Part print with two shaded views. Sizes in mm from the minimum x, y, z corner. A direction names the side the tool comes from. Round coordinates to 2 decimals unless told otherwise and drop trailing zeros. Loops run counter-clockwise (first coordinate to the right, second up) from the corner with the lowest first, then second, coordinate; pieces in that order, holes last. Notation, with made-up numbers: M 9,66 L 54,66 A15 cw 54,72 Z; hole C 25.25,25.5 d2. An arc over 180 degrees is marked long. Answer as CSV lines item,"result". Start each with the question number.
Item 1: Which spindle directions (+Z, -Z, +X, -X, +Y, -Y) get a long thin tool onto all of the face, cutting with end or side? Do the marked faces 1 and 2. Say none if no direction does.
Item 2: Mould opens along Y. For the marked faces 3, 4, 5 and 6 say: pulls with the +Y half, pulls with the -Y half, needs draft (parallel to the pull), parting line crosses it, or undercut.
Item 3: Band-saw the part on C-C (z = 8.5). Give the cut face in (x, y), and give its area (3 significant figures).
Item 4: Band-saw the part on A-A (y = 66). Give the cut face in (x, z).
Item 5: Band-saw the part on B-B (x = 5). Give the cut face in (y, z).
Item 6: Wall check: line 1 (Y direction, x = 77, z = 15.25); line 2 (X direction, y = 46, z = 10.25); line 3 (Y direction, x = 30.5, z = 2.25). Give the ranges that are in metal, low to high.
Item 7: Band-saw the part on D-D (x = 68.5). Give the cut face in (y, z).
Item 8: Drop a flat-ended pin along its axis: pin 1 Ø3.5 at (x, y) = (5, 5) entering from +Z. Give the stop position or say it passes through.
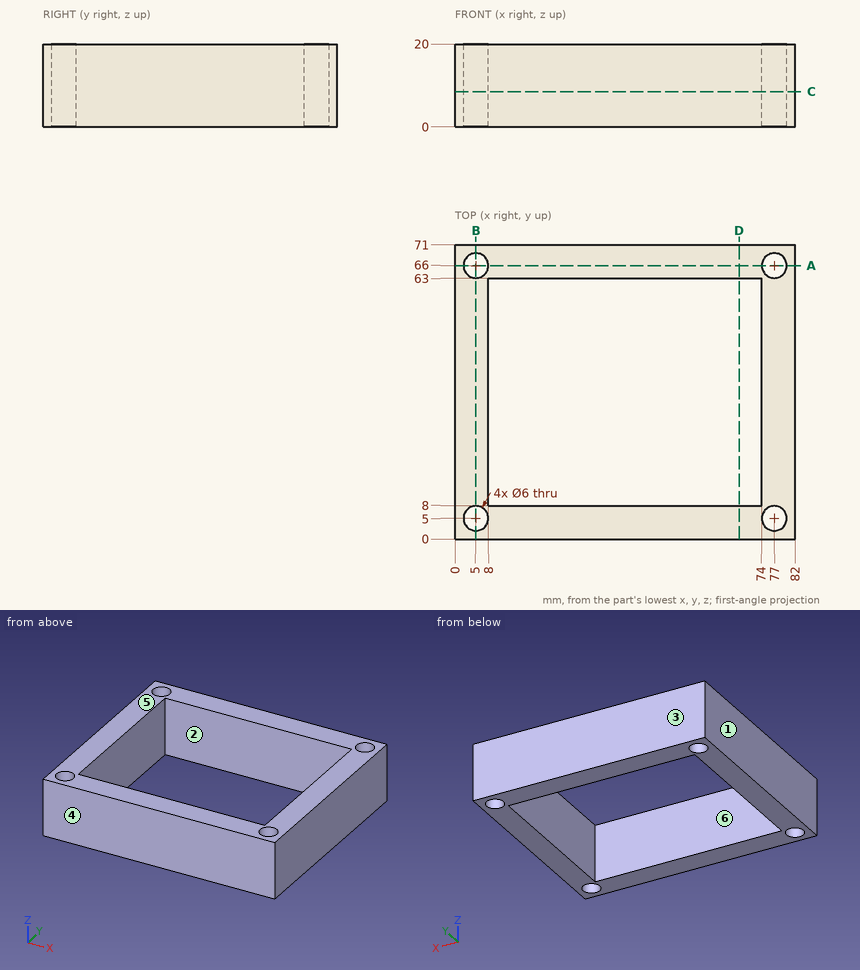
Answer block:
1,face 1,"+Z, -Z, -X, +Y, -Y"
1,face 2,"+Z, -Z"
2,face 3,"pulls with the +Y half"
2,face 4,"pulls with the -Y half"
2,face 5,"needs draft"
2,face 6,"undercut"
3,outline,"M 0,0 L 82,0 L 82,71 L 0,71 Z; hole C 5,5 d6; hole C 5,66 d6; hole M 8,8 L 74,8 L 74,63 L 8,63 Z; hole C 77,5 d6; hole C 77,66 d6"
3,area,"2,080 mm^2"
4,outline,"M 0,0 L 2,0 L 2,20 L 0,20 Z; M 8,0 L 74,0 L 74,20 L 8,20 Z; M 80,0 L 82,0 L 82,20 L 80,20 Z"
5,outline,"M 0,0 L 2,0 L 2,20 L 0,20 Z; M 8,0 L 63,0 L 63,20 L 8,20 Z; M 69,0 L 71,0 L 71,20 L 69,20 Z"
6,line 1,"y = 0 to 2, 8 to 63, 69 to 71"
6,line 2,"x = 0 to 8, 74 to 82"
6,line 3,"y = 0 to 8, 63 to 71"
7,outline,"M 0,0 L 8,0 L 8,20 L 0,20 Z; M 63,0 L 71,0 L 71,20 L 63,20 Z"
8,pin 1,"passes through"
